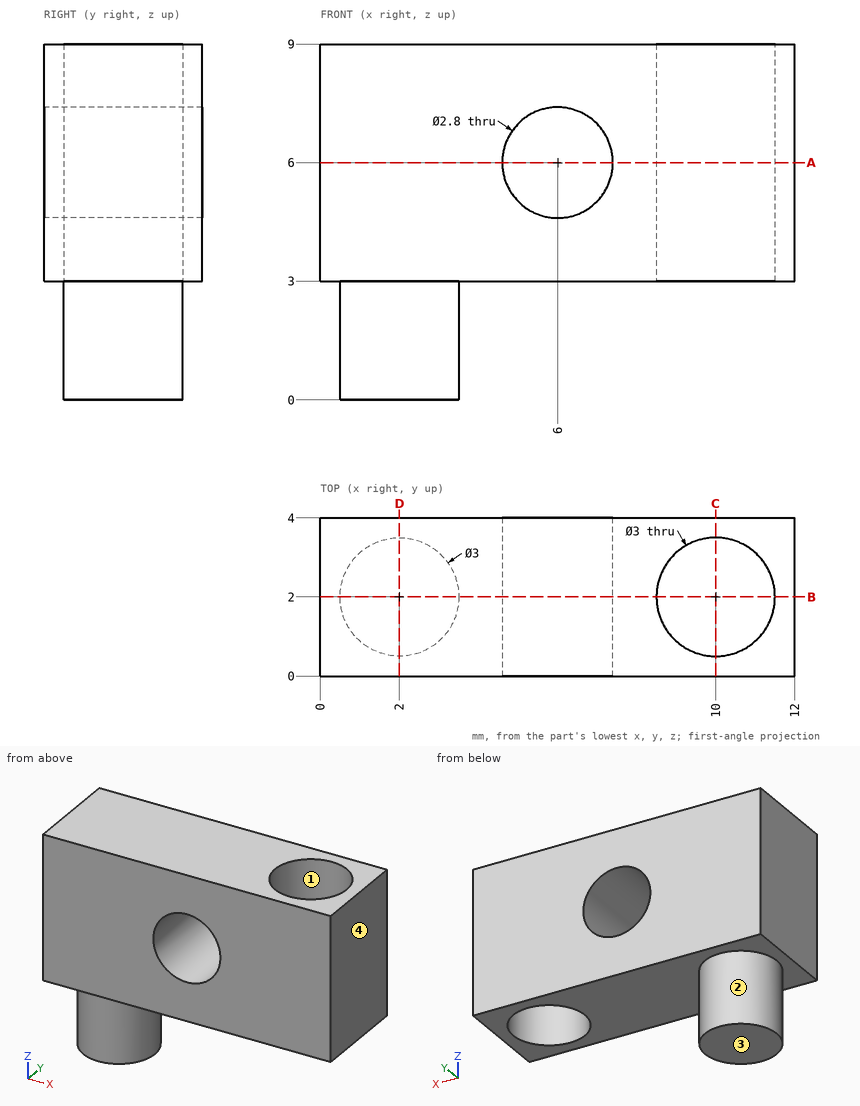
Part print with two shaded views. Sizes in mm from the minimum x, y, z corner. Round coordinates to 2 decimals unless told otherwise and drop trailing zeros. Order: outer loops, then holes, each group sorted by start corner. A loop starts at its lowest first (then second) coordinate and runs counter-clockwise, first axis right, second up.
(1) Pull direction X, two halves, no side cores. Call the marked faces 1, 2, 3 and 4: released by +X, released by -X, zero draft, split by the parting line, or undercut.
(2) Drill centre lines: line 1 (Z direction, x = 6, y = 2); line 2 (Y direction, x = 10, z = 4.4); line 3 (X direction, y = 1.5, z = 5). Where is each one in solid material? Low to high.
(3) Pin check, flat tip, straight feed: pin 1 (2 mm diameter, centred on x = 6.5, y = 1.5, fed in from -Z). Stop position of the tip, or through.
(4) Band-saw the part on D-D (x = 2). List the corners of the cut face in (y, z).
(5) Band-saw the part on A-A (z = 6). List the corners of the cut face in (x, y), then the cut area to 3 significant figures.
(6) Band-saw the part on B-B (y = 2). List the corners of the cut face in (x, z).
(7) Band-saw the part on C-C (x = 10). List the corners of the cut face in (y, z).
Verdict:
1. face 1: undercut
1. face 2: split by the parting line
1. face 3: zero draft
1. face 4: released by +X
2. line 1: z = 3 to 4.6, 7.4 to 9
2. line 2: y = 0 to 0.5, 3.5 to 4
2. line 3: x = 0 to 5.02, 6.98 to 8.59, 11.41 to 12
3. pin 1: stops at z = 3
4. outline: (0, 3) - (0.5, 3) - (0.5, 0) - (3.5, 0) - (3.5, 3) - (4, 3) - (4, 9) - (0, 9) - close
5. outline: (0, 0) - (4.6, 0) - (4.6, 4) - (0, 4) - close; (7.4, 0) - (12, 0) - (12, 4) - (7.4, 4) - close; hole circle Ø3 at (10, 2)
5. area: 29.7 mm2
6. outline: (0, 3) - (0.5, 3) - (0.5, 0) - (3.5, 0) - (3.5, 3) - (8.5, 3) - (8.5, 9) - (0, 9) - close; (11.5, 3) - (12, 3) - (12, 9) - (11.5, 9) - close; hole circle Ø2.8 at (6, 6)
7. outline: (0, 3) - (0.5, 3) - (0.5, 9) - (0, 9) - close; (3.5, 3) - (4, 3) - (4, 9) - (3.5, 9) - close
